```python
from build123d import *

# Parameters (mm, degrees)
F2_R           = 1.5875
F3_W           = 25.4
F3_H           = 15.875
F4_DEPTH       = 12.7
F6_D           = 1.5875
F6_DEPTH       = 19.05
F6_CBORE_D     = 3.175
F6_CBORE_DEPTH = 6.35


with BuildPart() as f1:
    # F0 (on Front) → F1 (revolve)
    with BuildSketch(Plane.XZ):
        Polygon((7.9375, 12.7), (0, 12.7), (0, 0), (6.35, 0), (7.9375, 4.36162), align=None)
    revolve(axis=Axis((0, 0, 6.35), (0, 0, 1)))

    # F2
    f2_edges = [f1.edges().sort_by_distance(p)[0] for p in [
        (-6.35, 0, 0),
        (-7.9375, 0, 4.36162),
    ]]
    fillet(f2_edges, radius=F2_R)

    # F3 (on Front) → F4 (cut, symmetric)
    with BuildSketch(Plane.XZ):
        with Locations((0, 12.7)):
            Rectangle(F3_W, F3_H)
    extrude(amount=F4_DEPTH, both=True, mode=Mode.SUBTRACT)

    # F6
    with Locations(Plane(origin=(0, 0, 0), x_dir=(1, 0, 0), z_dir=(0, 0, -1))):
        with Locations((0, 0)):
            CounterBoreHole(F6_D / 2, F6_CBORE_D / 2, F6_CBORE_DEPTH, depth=F6_DEPTH)


solid = f1.part
```
Can you work these out from the model? Positions are in its coordinate system, mm. Coordinates: 2 decimals unless noted, no trailing zeros. Write each loop counter-clockwise with the first axis right and the second up, starting at its lowest first coordinate (ties: lowest second). Pieces come first, ordered by that corner, then holes. Notation, with made-up numbers: M 51,-4 L 108,-4 A16 cw 108,16 Z; hole C -2.5,42.5 d11. An arc over 180 degrees is marked long. Write item = value, one per line. Start each with the question number.
Q1. Thinking about a two-plate mould opening in X: for faces 1 (the face through (-0.34, 1.55, 2.35)), 2 (the face through (3.138, -6.033, 1.236)), 3 (the face through (2, 0, 4.762)), which applies, released by +X, released by -X, zero draft, split by the parting line, or undercut?
Q2. If I drill on L1, parallel to Y at x = 0.25, z = 0.95; L2, parallel to X at y = 1.25, z = 2.6; L3, parallel to Y at x = 0.25, z = 0.6, over which ranges is the centre line in solid material (lowest first)? Write a range as [from, to].
Q3. I'm going to push flat-ended pins straight in: pin 1 (1.5 mm diameter, centred on y = -5, z = 3, fed in from -X); pin 2 (1 mm diameter, centred on x = 3, z = 4, fed in from +Y); pin 3 (2 mm diameter, centred on x = -3.5, z = 1.5, fed in from +Y). Where does each tip first touch, or does it pass through?
Q4. If we section it at B-B, the plane z = 0.8: Write out the boundary of the cut face in (x, y) (1 decimal), then the cut area to 3 significant figures.
Q5. If we section it at A-A, the plane z = 2.05: Write out the boundary of the cut face in (x, y) (1 decimal), then the cut area to 3 significant figures.
Check sheet entries:
q1.face_1 = undercut
q1.face_2 = split by the parting line
q1.face_3 = zero draft
q2.L1 = [-6.69, -1.57], [1.57, 6.69]
q2.L2 = [-7.19, -0.98], [0.98, 7.19]
q2.L3 = [-6.48, -1.57], [1.57, 6.48]
q3.pin_1 = -6.21
q3.pin_2 = 7.46
q3.pin_3 = 6.59
q4.outline = C 0,0 d13.2; hole C 0,0 d3.2
q4.area = 130 mm²
q5.outline = C 0,0 d14.2; hole C 0,0 d3.2
q5.area = 150 mm²
